from build123d import *

# Parameters (mm, degrees)
SKETCH_2_R          = 1.785
SKETCH_2_R_2        = 1.27
EXTRUDE_2_DEPTH     = 8.13
FILLET_1_R          = 0.5
FILLET_2_R          = 0.5
FILLET_3_R          = 0.5
SKETCH_5_R          = 1.785
CUT_EXTRUDE_1_DEPTH = 18
CHAMFER_1_SIZE      = 0.75


with BuildPart() as part:
    # Эскиз1 → Повернуть1 (revolve)
    with BuildSketch(Plane(origin=(0, 0, 0), x_dir=(0, 0, -1), z_dir=(1, 0, 0))):
        with BuildLine():
            Line((7.81, 0), (7.81, 38.61))
            Line((7.81, 38.61), (0, 38.61))
            Line((0, 38.61), (0, -34.919667125))
            Line((0, -34.919667125), (2.135124109, -34.919667125))
            Line((2.135124109, -34.919667125), (2.913509872, -34.919667125))
            ThreePointArc((2.913509872, -34.919667125), (3.658458343, -34.255552274), (3.935124109, -33.296671252))
            Line((3.935124109, -33.296671252), (3.935124109, -13.000030341))
            ThreePointArc((3.935124109, -13.000030341), (4.018123706, -11.486391771), (4.28668668, -9.994458602))
            Line((4.28668668, -9.994458602), (6.73, 0))
            Line((6.73, 0), (7.81, 0))
        make_face()
    revolve(axis=Axis((0, -34.919667125, 0), (0, 1, 0)))

    # Эскиз2 → Бобышка-Вытянуть2 (add)
    with BuildSketch(Plane(origin=(0, 38.61, 0), x_dir=(1, 0, 0), z_dir=(0, 1, 0))):
        with Locations((0, 3.18)):
            Circle(SKETCH_2_R)
        with Locations((0, 3.18)):
            Circle(SKETCH_2_R_2, mode=Mode.SUBTRACT)
    extrude(amount=EXTRUDE_2_DEPTH)

    # Скругление1
    fillet_1_edges = [part.edges().sort_by_distance(p)[0] for p in [
        (-1.785, 46.74, -3.18),
    ]]
    fillet(fillet_1_edges, radius=FILLET_1_R)

    # Скругление2
    fillet_2_edges = [part.edges().sort_by_distance(p)[0] for p in [
        (-1.785, 38.61, -3.18),
    ]]
    fillet(fillet_2_edges, radius=FILLET_2_R)

    # Скругление3
    fillet_3_edges = [part.edges().sort_by_distance(p)[0] for p in [
        (0, 38.61, 7.81),
        (0, 0, 7.81),
    ]]
    fillet(fillet_3_edges, radius=FILLET_3_R)

    # Эскиз5 → Вырез-Вытянуть1 (cut)
    with BuildSketch(Plane(origin=(0, 39.61, 0), x_dir=(1, 0, 0), z_dir=(0, 1, 0))):
        with Locations((0, -3.18)):
            Circle(SKETCH_5_R)
    extrude(amount=-CUT_EXTRUDE_1_DEPTH, mode=Mode.SUBTRACT)

    # Фаска1
    chamfer_1_edges = [part.edges().sort_by_distance(p)[0] for p in [
        (-1.785, 38.61, 3.18),
    ]]
    chamfer(chamfer_1_edges, length=CHAMFER_1_SIZE)


solid = part.part
Geometry: final body of the model. Coordinates: model frame, mm. A direction names the side the tool comes from. Round coordinates to 2 decimals unless told otherwise and drop trailing zeros. Write each loop counter-clockwise with the first axis right and the second up, starting at its lowest first coordinate (ties: lowest second). Pieces come first, ordered by that corner, then holes. Notation, with made-up numbers: M 73.25,16.25 L 102.25,16.25 A20 ccw 102.25,31.25 Z; hole C 20,-16.75 d3. An arc over 180 degrees is marked long. Write item = value, one per line.
Item 1: Pull-direction query (Z, two-part tool) for faces 4 (the face through (-0.39, 42.63, -1.44)), 5 (the face through (5, 0, 5)), 6 (the face through (-0.17, 42.62, -4.44)); classes: pulls with the +Z half, pulls with the -Z half, needs draft (parallel to the pull), parting line crosses it, or undercut.
Findings:
face_4 = parting line crosses it
face_5 = needs draft
face_6 = undercut
Item 2: Access query for faces 1 (the face through (0, 21.61, 3)), 2 (the face through (3.842, -23.006, 0.853)), 3 (the face through (0, -34.92, 0)). Directions: +Z, -Z, +X, -X, +Y, -Y. A direction counts if a zero-diameter tool reaches every point of the face in a straight line with its end or side. Return the directions, or none.
Findings:
face_1 = +Y
face_2 = -Y
face_3 = +Z, -Z, +X, -X, -Y
Item 3: Pin query (flat end, axial travel): P1, Ø1, axis at y = 1, z = -1, coming from the +X side; P2, Ø8, axis at x = -5, y = -3, coming from the -Z side; P3, Ø1, axis at y = 2, z = 5, coming from the -X side. Return the tip coordinate at first contact, or that it passes through.
Findings:
P1 = 7.79
P2 = -7.27
P3 = -6.38
Item 4: Section query A-A on y = 25. Return loops of the section in (x, z) (3 decimals), then the cut area to 3 significant figures.
Findings:
outline = C 0,0 d15.62; hole C 0,3.18 d3.57
area = 182 mm^2
Item 5: Material intervals for line 1 along Z through (x, y) = (0, 44.75) (3 decimals); line 2 along Z through (x, y) = (0, 26) (3 decimals); line 3 along X through (y, z) = (42, -3.18) (3 decimals), sorted ascending. Write a range as [from, to].
Findings:
line_1 = [-4.965, -4.45], [-1.91, -1.395]
line_2 = [-7.81, 1.395], [4.965, 7.81]
line_3 = [-1.785, -1.27], [1.27, 1.785]
